The figure shows three views and two pictorial views of one solid part (mm, origin at its lowest corner). Answer the questions. A direction names the side the tool comes from. Round coordinates to 2 decimals unless told otherwise and drop trailing zeros. Order: outer loops, then holes, each group sorted by start corner. A loop starts at its lowest first (then second) coordinate and runs counter-clockwise, first axis right, second up. Notation, with made-up numbers: (54, 77) - (113, 77) arc R19 ccw to (113, 93) - close; hole circle Ø6 at (28, 72). An arc over 180 degrees is marked (long way). One line per item, written item: value. Start each with the question number.
1. Section C-C, the plane x = 66 is taken. Give the vertices of the cut face in (y, z).
2. A tool of negligible diameter and unlimited length cuts with its end or side. For the marked faces 4, 5 and 6, from which of +Z, -Z, +X, -X, +Y, -Y can it reach the whole face along a straight path? Write none if from no direction.
3. Section A-A, the plane y = 50.8 is taken. Give the vertices of the cut face in (x, z).
4. Section D-D, the plane z = 38 is taken. Give the vertices of the cut face in (x, y) (1 decimal), then the cut area to 3 significant figures.
5. Flat-ended cylindrical pins translate along their axes: P1, Ø23, axis at x = 54.5, z = 53.5, coming from the +Y side; P2, Ø4, axis at x = 44.5, y = 9, coming from the +Z side; P3, Ø5, axis at x = 78, z = 20, coming from the -Y side. Find the tip coordinate at first contact, or state that the pin passes through.
6. Section B-B, the plane z = 58 is taken. Give the vertices of the cut face in (x, y).
7. For a pull along Y with two mould halves and no side action, classify the marked faces 1, 2 and 3 as released by +Y, released by -Y, zero draft, split by the parting line, or undercut.
8. Straight lines are drawn through the part: line 1 (Y direction, x = 38, z = 50); line 2 (Y direction, x = 38, z = 57); line 3 (Y direction, x = 53, z = 47). For each, find the intervals that lie inside material, in ascending order.
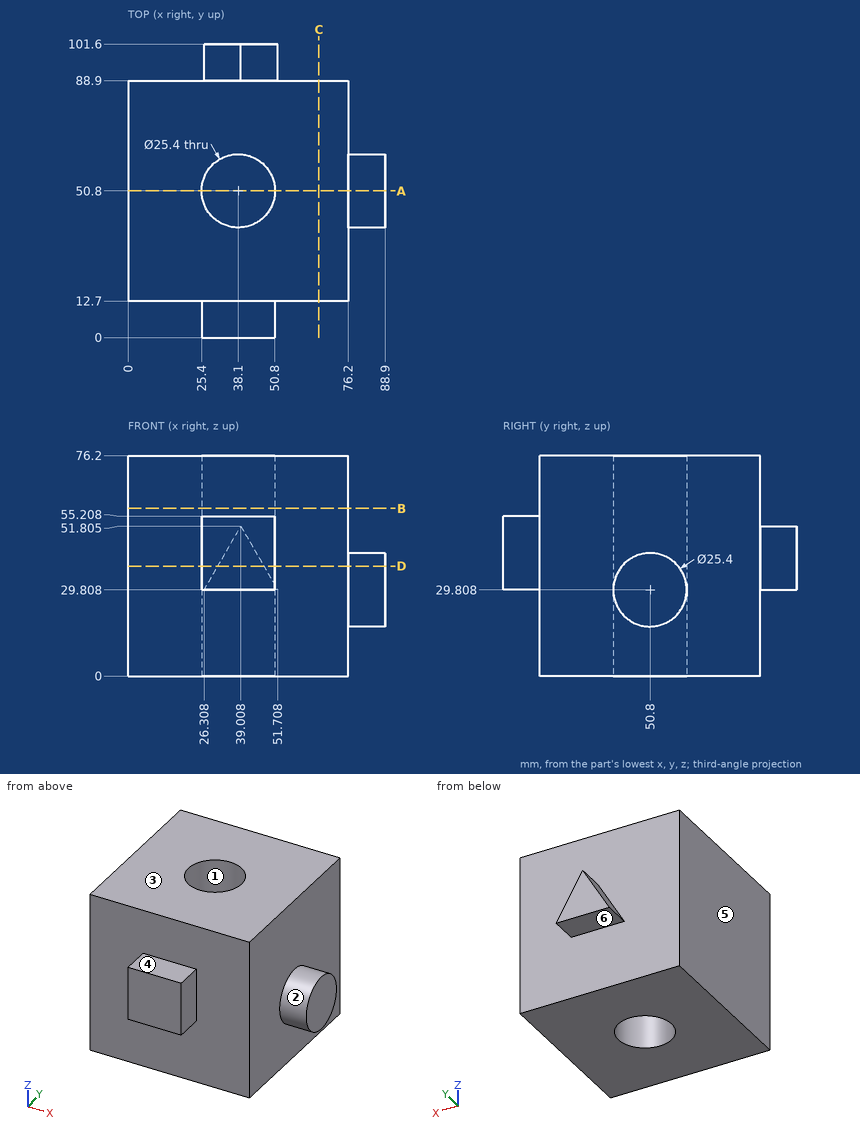
Answer list:
1. outline: (12.7, 0) - (88.9, 0) - (88.9, 76.2) - (12.7, 76.2) - close
2. face 4: +Z, +X, -X, -Y
2. face 5: +Z, -Z, -X, +Y, -Y
2. face 6: -Z, +X, -X, +Y
3. outline: (0, 0) - (25.4, 0) - (25.4, 76.2) - (0, 76.2) - close; (50.8, 0) - (76.2, 0) - (76.2, 17.11) - (88.9, 17.11) - (88.9, 42.51) - (76.2, 42.51) - (76.2, 76.2) - (50.8, 76.2) - close
4. outline: (0, 12.7) - (25.4, 12.7) - (25.4, 0) - (50.8, 0) - (50.8, 12.7) - (76.2, 12.7) - (76.2, 41.1) - (88.9, 41.1) - (88.9, 60.5) - (76.2, 60.5) - (76.2, 88.9) - (47, 88.9) - (47, 101.6) - (31, 101.6) - (31, 88.9) - (0, 88.9) - close; hole circle Ø25.4 at (38.1, 50.8)
4. area: 6,070 mm²
5. P1: stops at y = 88.9
5. P2: stops at z = 55.21
5. P3: stops at y = 12.7
6. outline: (0, 12.7) - (76.2, 12.7) - (76.2, 88.9) - (0, 88.9) - close; hole circle Ø25.4 at (38.1, 50.8)
7. face 1: undercut
7. face 2: split by the parting line
7. face 3: zero draft
8. line 1: y = 0 to 38.1, 63.5 to 101.6
8. line 2: y = 12.7 to 38.1, 63.5 to 88.9
8. line 3: y = 12.7 to 88.9
